Could you check a few things on this model? Use its own coordinates, in mm. Give positions to 0.01 mm unless a question says otherwise; leave off trailing zeros. Write each loop counter-clockwise with the first axis right and the second up, starting at its lowest first coordinate (ties: lowest second). Pieces come first, ordered by that corner, then holes. Notation, with made-up numbers: (0.25, 88) - (23.25, 88) arc R34 cw to (23.25, 118) - close; hole circle Ø5 at (67, 20). An arc over 180 degrees is marked (long way). Write item = value, one per line.
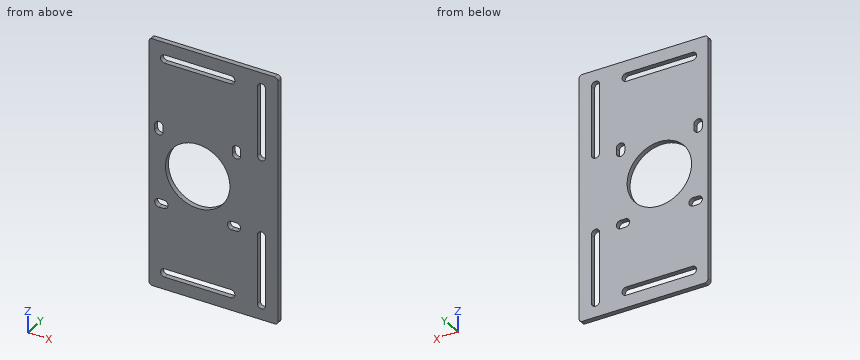
from build123d import *

# Parameters (mm, degrees)
SKETCH1_R           = 19.5
BOSS_EXTRUDE1_DEPTH = 3


with BuildPart() as part:
    # Sketch1 → Boss-Extrude1 (new body)
    with BuildSketch(Plane(origin=(0, 0, 0), x_dir=(1, 0, 0), z_dir=(0, 1, 0))):
        with BuildLine():
            Line((-37, 75), (37, 75))
            ThreePointArc((37, 75), (38.414213562, 74.414213562), (39, 73))
            Line((39, 73), (39, -73))
            ThreePointArc((39, -73), (38.414213562, -74.414213562), (37, -75))
            Line((37, -75), (-37, -75))
            ThreePointArc((-37, -75), (-38.414213562, -74.414213562), (-39, -73))
            Line((-39, -73), (-39, 73))
            ThreePointArc((-39, 73), (-38.414213562, 74.414213562), (-37, 75))
        make_face()
        with Locations(Location((-9.57, 0, 0), (0, 0, 270))):
            Circle(SKETCH1_R, mode=Mode.SUBTRACT)
        with BuildLine():
            Line((31.5, 65.876713653), (31.5, 24.123286347))
            ThreePointArc((31.5, 24.123286347), (29, 21.623286347), (26.5, 24.123286347))
            Line((26.5, 24.123286347), (26.5, 65.876713653))
            ThreePointArc((26.5, 65.876713653), (29, 68.376713653), (31.5, 65.876713653))
        make_face(mode=Mode.SUBTRACT)
        with BuildLine():
            Line((31.5, -65.876713653), (31.5, -24.123286347))
            ThreePointArc((31.5, -24.123286347), (29, -21.623286347), (26.5, -24.123286347))
            Line((26.5, -24.123286347), (26.5, -65.876713653))
            ThreePointArc((26.5, -65.876713653), (29, -68.376713653), (31.5, -65.876713653))
        make_face(mode=Mode.SUBTRACT)
        with BuildLine():
            Line((-29.57, 67.5), (10.43, 67.5))
            ThreePointArc((10.43, 67.5), (12.93, 65), (10.43, 62.5))
            Line((10.43, 62.5), (-29.57, 62.5))
            ThreePointArc((-29.57, 62.5), (-32.07, 65), (-29.57, 67.5))
        make_face(mode=Mode.SUBTRACT)
        with BuildLine():
            Line((-29.57, -67.5), (10.43, -67.5))
            ThreePointArc((10.43, -67.5), (12.93, -65), (10.43, -62.5))
            Line((10.43, -62.5), (-29.57, -62.5))
            ThreePointArc((-29.57, -62.5), (-32.07, -65), (-29.57, -67.5))
        make_face(mode=Mode.SUBTRACT)
        with BuildLine():
            Line((-33.028267466, 26.008267466), (-30.028267466, 26.008267466))
            ThreePointArc((-30.028267466, 26.008267466), (-27.478267466, 23.458267466), (-30.028267466, 20.908267466))
            Line((-30.028267466, 20.908267466), (-33.028267466, 20.908267466))
            ThreePointArc((-33.028267466, 20.908267466), (-35.578267466, 23.458267466), (-33.028267466, 26.008267466))
        make_face(mode=Mode.SUBTRACT)
        with BuildLine():
            Line((13.888267466, 26.008267466), (10.888267466, 26.008267466))
            ThreePointArc((10.888267466, 26.008267466), (8.338267466, 23.458267466), (10.888267466, 20.908267466))
            Line((10.888267466, 20.908267466), (13.888267466, 20.908267466))
            ThreePointArc((13.888267466, 20.908267466), (16.438267466, 23.458267466), (13.888267466, 26.008267466))
        make_face(mode=Mode.SUBTRACT)
        with BuildLine():
            Line((-35.578267466, -23.458267466), (-35.578267466, -20.458267466))
            ThreePointArc((-35.578267466, -20.458267466), (-33.028267466, -17.908267466), (-30.478267466, -20.458267466))
            Line((-30.478267466, -20.458267466), (-30.478267466, -23.458267466))
            ThreePointArc((-30.478267466, -23.458267466), (-33.028267466, -26.008267466), (-35.578267466, -23.458267466))
        make_face(mode=Mode.SUBTRACT)
        with BuildLine():
            Line((16.438267466, -23.458267466), (16.438267466, -20.458267466))
            ThreePointArc((16.438267466, -20.458267466), (13.888267466, -17.908267466), (11.338267466, -20.458267466))
            Line((11.338267466, -20.458267466), (11.338267466, -23.458267466))
            ThreePointArc((11.338267466, -23.458267466), (13.888267466, -26.008267466), (16.438267466, -23.458267466))
        make_face(mode=Mode.SUBTRACT)
    extrude(amount=BOSS_EXTRUDE1_DEPTH)


solid = part.part
1. I need wall thicknesses on line 1 (X direction, y = 1.55, z = 0); line 2 (X direction, y = 0.9, z = -51.5); line 3 (Z direction, x = -13, y = 0.3). Which ranges of each line are inside material? Lowest first, please.
Filled sheet:
line_1 = -39 to -29.07, 9.93 to 39
line_2 = -39 to 26.5, 31.5 to 39
line_3 = -75 to -67.5, -62.5 to -19.2, 19.2 to 62.5, 67.5 to 75
2. If we section it at A-A, the plane x = -9.57: Please give me the cut outline in (y, z), and give its area (3 significant figures).
Filled sheet:
outline = (0, -75) - (3, -75) - (3, -67.5) - (0, -67.5) - close; (0, -62.5) - (3, -62.5) - (3, -19.5) - (0, -19.5) - close; (0, 19.5) - (3, 19.5) - (3, 62.5) - (0, 62.5) - close; (0, 67.5) - (3, 67.5) - (3, 75) - (0, 75) - close
area = 303 mm2
3. If we section it at B-B, the plane z = -37.5: Please give me the cut outline in (x, y).
Filled sheet:
outline = (-39, 0) - (26.5, 0) - (26.5, 3) - (-39, 3) - close; (31.5, 0) - (39, 0) - (39, 3) - (31.5, 3) - close
4. If we section it at C-C, the plane x = 29: Please give me the cut outline in (y, z).
Filled sheet:
outline = (0, -75) - (3, -75) - (3, -68.38) - (0, -68.38) - close; (0, -21.62) - (3, -21.62) - (3, 21.62) - (0, 21.62) - close; (0, 68.38) - (3, 68.38) - (3, 75) - (0, 75) - close
5. If we section it at D-D, the plane z = 0: Please give me the cut outline in (x, y).
Filled sheet:
outline = (-39, 0) - (-29.07, 0) - (-29.07, 3) - (-39, 3) - close; (9.93, 0) - (39, 0) - (39, 3) - (9.93, 3) - close
